Could you check a few things on this model? Use its own coordinates, in mm. A direction names the side the tool comes from. Round coordinates to 2 decimals unless told otherwise and drop trailing zeros. Loops run counter-clockwise (first coordinate to the right, second up) from the corner with the lowest first, then second, coordinate; pieces in that order, holes last.
from build123d import *

# Parameters (mm, degrees)
ESQUISSE1_W             = 6.35
ESQUISSE1_H             = 6.35
BOSS_EXTRU_1_DEPTH      = 13
BOSS_EXTRU_2_DEPTH      = 15
BOSS_EXTRU_2_DEPTH_BACK = 28
ESQUISSE2_R             = 3
CONG_1_R                = 0.5


with BuildPart() as part:
    # Esquisse1 → Boss.-Extru.1 (new body)
    with BuildSketch(Plane(origin=(0, 0, 0), x_dir=(1, 0, 0), z_dir=(0, 1, 0))):
        with Locations((3.175, 3.175)):
            Rectangle(ESQUISSE1_W, ESQUISSE1_H)
    extrude(amount=BOSS_EXTRU_1_DEPTH)

    # Esquisse2 → Boss.-Extru.2 (add, two sides: drawn at the far end of the back side and taken through both)
    with BuildSketch(Plane(origin=(0, 13, 0), x_dir=(1, 0, 0), z_dir=(0, 1, 0)).offset(-BOSS_EXTRU_2_DEPTH_BACK)):
        with Locations(Location((3.175, 3.175, 0), (0, 0, 270))):
            Circle(ESQUISSE2_R)
    extrude(amount=BOSS_EXTRU_2_DEPTH + BOSS_EXTRU_2_DEPTH_BACK)

    # Congé1
    cong_1_edges = [part.edges().sort_by_distance(p)[0] for p in [
        (0, 6.5, -6.35),
        (6.35, 6.5, -6.35),
        (6.35, 6.5, 0),
        (0, 6.5, 0),
    ]]
    fillet(cong_1_edges, radius=CONG_1_R)


solid = part.part
Item 1: For faces 1 (the cylindrical face through (3.31, -7.6, -6.17)), 2 (the cylindrical face through (3.31, 20.39, -6.17)), 3 (the flat face through (3, 28, -3)), which set-ups out of +Z, -Z, +X, -X, +Y, -Y let a thin tool reach every point of the face, with its end or its side?
Results list:
face 1: -Y
face 2: +Y
face 3: +Z, -Z, +X, -X, +Y
Item 2: Will this pin go through, and if not, where does the flat tip stop? pin 1 (3 mm diameter, centred on x = 3.5, y = -3.5, fed in from +Z) (3 decimals).
Results list:
pin 1: stops at z = -0.175
Item 3: If we section it at A-A, the plane x = 1.5: Please give me the cut outline in (y, z).
Results list:
outline: (-15, -5.66) - (0, -5.66) - (0, -6.35) - (13, -6.35) - (13, -5.66) - (28, -5.66) - (28, -0.69) - (13, -0.69) - (13, 0) - (0, 0) - (0, -0.69) - (-15, -0.69) - close
Item 4: If I drill on line 1 along Y through (x, z) = (5.5, -5.75); line 2 along Z through (x, y) = (3, 14); line 3 along Z through (x, y) = (1, 24), over which ranges is the centre line in solid material (lowest first)?
Results list:
line 1: y = 0 to 13
line 2: z = -6.17 to -0.18
line 3: z = -5.24 to -1.11
Item 5: If we section it at B-B, the plane z = -5: Please give me the cut outline in (x, y).
Results list:
outline: (0, 0) - (0.79, 0) - (0.79, -15) - (5.56, -15) - (5.56, 0) - (6.35, 0) - (6.35, 13) - (5.56, 13) - (5.56, 28) - (0.79, 28) - (0.79, 13) - (0, 13) - close
Item 6: If we section it at C-C, the plane y = -5.5: Please give me the cut outline in (x, z) (3 decimals), then the cut area to 3 significant figures.
Results list:
outline: circle Ø6 at (3.175, -3.175)
area: 28.3 mm2
